Autodesk Inventor part; units mm, degrees
ref_plane "YZ Plane" through (0, 0, 0) normal (1, 0, 0) x (0, 1, 0)
ref_plane "XZ Plane" through (0, 0, 0) normal (0, 1, 0) x (-1, 0, 0)
ref_plane "XY Plane" through (0, 0, 0) normal (0, 0, 1) x (1, 0, 0)
sketch "Sketch1" plane through (0, 0, 0) normal (1, 0, 0) x (0, 1, 0)
  line L0 (-4.5, 10) -> (4.5, 10)
  line L1 (4.5, 10) -> (4.5, -10)
  line L2 (4.5, -10) -> (-4.5, -10)
  line L3 (-4.5, -10) -> (-4.5, 10)
  line L4 (-4.5, 10) -> (4.5, -10) construction
  line L5 (4.5, 10) -> (-4.5, -10) construction
  circle A0 centre (0, 0) radius 1.65
  point P0 (0, 0)
  dimension "d0" = 9
  dimension "d1" = 20
  dimension "d2" = 3.3
extrude "Extrusion1" add sketch "Sketch1" along normal blind 4.3
properties part number "GPU Clamp"
The listing builds one solid part. Answer for the finished solid, in the listing's coordinates (mm). Round coordinates to 2 decimals unless told otherwise and drop trailing zeros. Write each loop counter-clockwise with the first axis right and the second up, starting at its lowest first coordinate (ties: lowest second). Pieces come first, ordered by that corner, then holes. Notation, with made-up numbers: M 61,24.25 L 95,24.25 A22 cw 95,37.25 Z; hole C -10.75,72 d11. An arc over 180 degrees is marked long. Write each question's results on one line, items separated by ' | '. Start each with the question number.
(1) The part is cut by section B-B, the plane z = 0. Write down the section's boundary in (x, y), and give its area (3 significant figures).
(2) The part is cut by section C-C, the plane x = 3.9. Write down the section's boundary in (y, z), and give its area (3 significant figures).
(3) The part is cut by section A-A, the plane y = 0. Write down the section's boundary in (x, z), and give its area (3 significant figures).
(4) Determine the mould class of faces 1 (the flat face through (2, -4.5, 0)), 2 (the cylindrical face through (2.12, -1.216, -1.115)), 3 (the flat face through (2, 0, 10)), 4 (the flat face through (2, 4.5, 0)) for opening direction Y: +Y half, -Y half, draft (parallel to the pull), parting line (faces both ways), or undercut.
(5) Find the intervals of material crossed by line 1 (Z direction, x = 2, y = 0); line 2 (Z direction, x = 2.85, y = 1.5); line 3 (Y direction, x = 3, z = -1.5), in increasing order.
Worked answers:
1) outline: M 0,-4.5 L 4.3,-4.5 L 4.3,-1.65 L 0,-1.65 Z; M 0,1.65 L 4.3,1.65 L 4.3,4.5 L 0,4.5 Z | area: 24.5 mm²
2) outline: M -4.5,-10 L 4.5,-10 L 4.5,10 L -4.5,10 Z; hole C 0,0 d3.3 | area: 171 mm²
3) outline: M 0,-10 L 4.3,-10 L 4.3,-1.65 L 0,-1.65 Z; M 0,1.65 L 4.3,1.65 L 4.3,10 L 0,10 Z | area: 71.8 mm²
4) face 1: -Y half | face 2: undercut | face 3: draft | face 4: +Y half
5) line 1: z = -10 to -1.65, 1.65 to 10 | line 2: z = -10 to -0.69, 0.69 to 10 | line 3: y = -4.5 to -0.69, 0.69 to 4.5
